The listing builds one solid part. Answer for the finished solid, in the listing's coordinates (mm). Round coordinates to 2 decimals unless told otherwise and drop trailing zeros. Write each loop counter-clockwise with the first axis right and the second up, starting at its lowest first coordinate (ties: lowest second). Pieces come first, ordered by that corner, then holes. Notation, with made-up numbers: (60.5, -4.75) - (70.5, -4.75) arc R25 ccw to (70.5, 16.25) - close; hole circle Ø3 at (33.5, 72). An arc over 180 degrees is marked (long way). Answer in a Markdown table with one row per item.
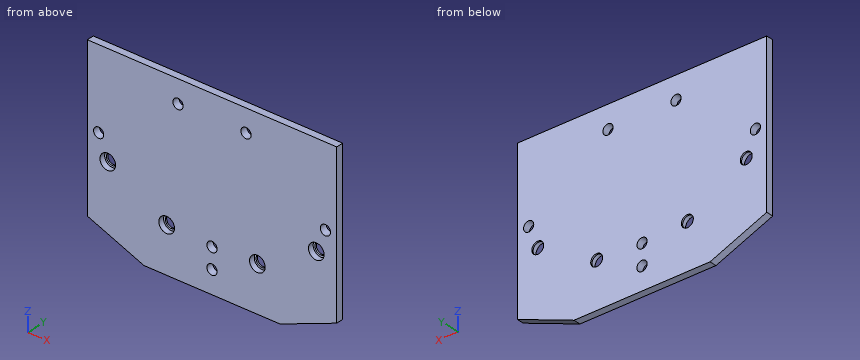
from build123d import *

# Parameters (mm, degrees)
BOSS_EXTRUDE1_DEPTH   = 1.5875
F_1_0MM_DOWEL_HOLE1_D = 5.25
SKETCH6_R             = 3.45
CUT_EXTRUDE2_DEPTH    = 2.5
M4_CLEARANCE_HOLE1_D  = 4.5
M4_CLEARANCE_HOLE2_D  = 4.5
M4_CLEARANCE_HOLE3_D  = 4.5


with BuildPart() as part:
    # Sketch1 → Boss-Extrude1 (new body, symmetric)
    with BuildSketch(Plane(origin=(0, 0, 0), x_dir=(1, 0, 0), z_dir=(0, 1, 0))):
        Polygon((-55, 15), (-30, 25), (30, 25), (55, 15), (55, -55), (-55, -55), align=None)
    extrude(amount=BOSS_EXTRUDE1_DEPTH, both=True)

    # Ø1.0mm Dowel Hole1 (through all)
    with Locations(Plane(origin=(0, 1.5875, 0), x_dir=(1, 0, 0), z_dir=(0, 1, 0))):
        with Locations((-20, 5), (20, 5), (45.980762114, -10), (-45.980762114, -10)):
            Hole(F_1_0MM_DOWEL_HOLE1_D / 2)

    # Sketch6 → Cut-Extrude2 (cut)
    with BuildSketch(Plane.XZ.offset(1.5875)):
        with Locations((-45.980762114, 10)):
            Circle(SKETCH6_R)
        with Locations((-20, -5)):
            Circle(SKETCH6_R)
        with Locations((20, -5)):
            Circle(SKETCH6_R)
        with Locations((45.980762114, 10)):
            Circle(SKETCH6_R)
    extrude(amount=-CUT_EXTRUDE2_DEPTH, mode=Mode.SUBTRACT)

    # M4 Clearance Hole1 (through all)
    with Locations(Plane(origin=(0, -1.5875, 0), x_dir=(-1, 0, 0), z_dir=(0, -1, 0))):
        with Locations((0, 15), (0, 6)):
            Hole(M4_CLEARANCE_HOLE1_D / 2)

    # M4 Clearance Hole2 (through all)
    with Locations(Plane(origin=(0, 1.5875, 0), x_dir=(1, 0, 0), z_dir=(0, 1, 0))):
        with Locations((-15, -45), (15, -45)):
            Hole(M4_CLEARANCE_HOLE2_D / 2)

    # M4 Clearance Hole3 (through all)
    with Locations(Plane(origin=(0, 1.5875, 0), x_dir=(1, 0, 0), z_dir=(0, 1, 0))):
        with Locations((-50, -20), (50, -20)):
            Hole(M4_CLEARANCE_HOLE3_D / 2)


solid = part.part
(1) Find the intervals of material crossed by line 1 (X direction, y = 1.2, z = 10); line 2 (Z direction, x = -20, y = -0.7); line 3 (X direction, y = -0.05, z = 45), in increasing order.
Checked values:
| item | result |
|---|---|
| line 1 | x = -55 to -48.61, -43.36 to 43.36, 48.61 to 55 |
| line 2 | z = -25 to -8.45, -1.55 to 55 |
| line 3 | x = -55 to -17.25, -12.75 to 12.75, 17.25 to 55 |
(2) Flat-ended cylindrical pins translate along their axes: pin 1 (6 mm diameter, centred on x = -45.98, z = 10, fed in from +Y); pin 2 (1.5 mm diameter, centred on x = -42, y = 1, fed in from -Z); pin 3 (3.5 mm diameter, centred on x = 50, z = 20, fed in from -Y); pin 4 (2 mm diameter, centred on x = 47.5, z = 11.5, fed in from -Y). Find the tip coordinate at first contact, or state that the pin passes through.
Checked values:
| item | result |
|---|---|
| pin 1 | stops at y = 1.59 |
| pin 2 | stops at z = -20.5 |
| pin 3 | passes through |
| pin 4 | stops at y = 0.91 |
(3) Section B-B (z = 20) is taken. Give the vertices of the cut face in (x, y).
Checked values:
| item | result |
|---|---|
| outline | (-55, -1.59) - (-52.25, -1.59) - (-52.25, 1.59) - (-55, 1.59) - close; (-47.75, -1.59) - (47.75, -1.59) - (47.75, 1.59) - (-47.75, 1.59) - close; (52.25, -1.59) - (55, -1.59) - (55, 1.59) - (52.25, 1.59) - close |
(4) Section D-D (x = 0) is taken. Give the vertices of the cut face in (y, z), and give its area (3 significant figures).
Checked values:
| item | result |
|---|---|
| outline | (-1.59, -25) - (1.59, -25) - (1.59, -17.25) - (-1.59, -17.25) - close; (-1.59, -12.75) - (1.59, -12.75) - (1.59, -8.25) - (-1.59, -8.25) - close; (-1.59, -3.75) - (1.59, -3.75) - (1.59, 55) - (-1.59, 55) - close |
| area | 225 mm2 |
(5) Section C-C (y = 0.1) is taken. State how many separate pieces and enclosed holes the cut face has, and give its area (4 significant figures).
Checked values:
| item | result |
|---|---|
| separate pieces | 1 |
| enclosed holes | 10 |
| area | 8,305 mm2 |
